The figure shows three views and two pictorial views of one solid part (mm, origin at its lowest corner). Answer the questions. A direction names the side the tool comes from. Give positions to 0.01 mm unless a question says otherwise; leave off trailing zeros. Order: outer loops, then holes, each group sorted by start corner. A loop starts at its lowest first (then second) coordinate and runs counter-clockwise, first axis right, second up. Notation, with made-up numbers: (82.5, -7.5) -> (124.5, -7.5) arc R17 cw to (124.5, 4.5) -> close; hole circle Ø4 at (23, 25.25). An arc over 180 degrees is marked (long way). Use one line per item in the form item = value.
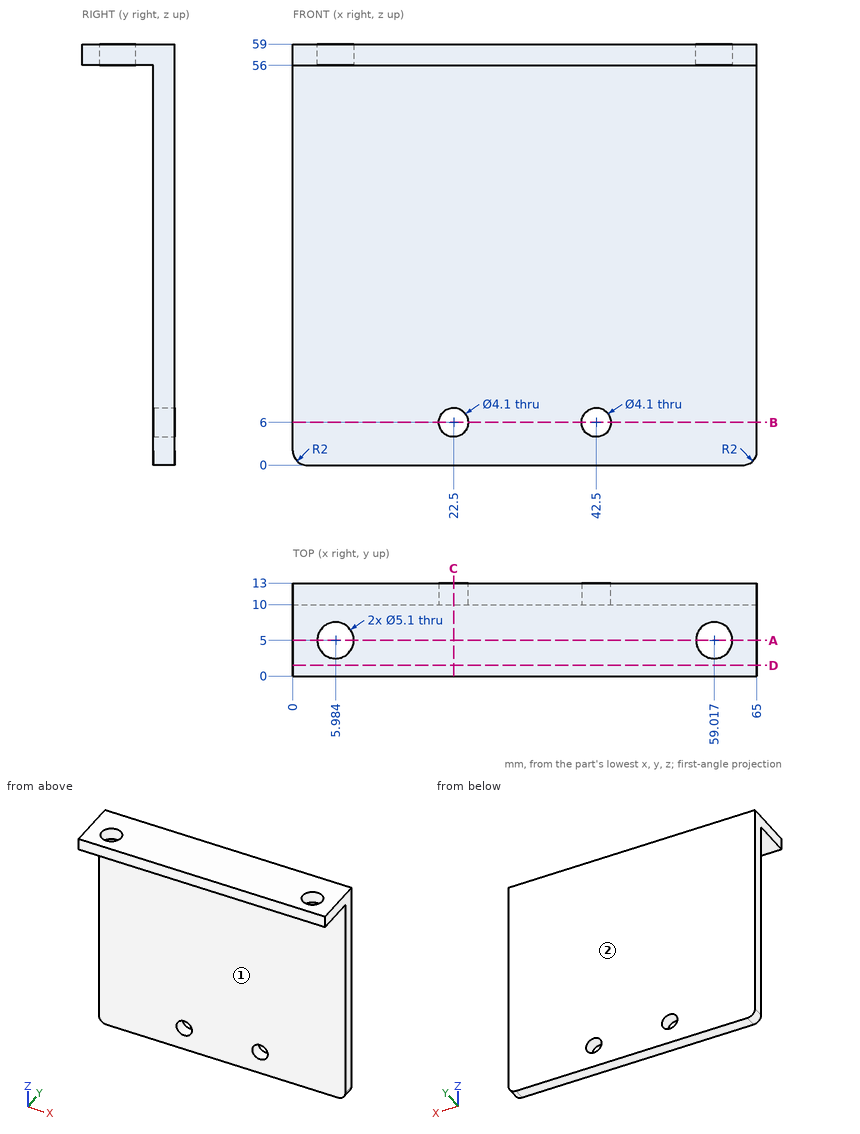
Item 1: The part is cut by section B-B on z = 6. Give the vertices of the cut face in (x, y).
Checks:
outline = (0, 10) -> (20.45, 10) -> (20.45, 13) -> (0, 13) -> close; (24.55, 10) -> (40.45, 10) -> (40.45, 13) -> (24.55, 13) -> close; (44.55, 10) -> (65, 10) -> (65, 13) -> (44.55, 13) -> close
Item 2: Given pin 1 Ø6 at (x, z) = (36.5, 50.5) entering from -Y; pin 2 Ø2 at (x, y) = (26.5, 2) entering from -Z, each flat-ended and moving along its own axis, determine where each tip first touches the part or whether it passes through.
Checks:
pin_1 = 10
pin_2 = 56
Item 3: The part is cut by section D-D on y = 1.5. Give the vertices of the cut face in (x, z).
Checks:
outline = (0, 56) -> (65, 56) -> (65, 59) -> (0, 59) -> close
Item 4: The part is cut by section C-C on x = 22.5. Give the vertices of the cut face in (y, z).
Checks:
outline = (0, 56) -> (10, 56) -> (10, 8.05) -> (13, 8.05) -> (13, 59) -> (0, 59) -> close; (10, 0) -> (13, 0) -> (13, 3.95) -> (10, 3.95) -> close
Item 5: Straight lines are drawn through the part: L1, parallel to Z at x = 22.5, y = 11.5; L2, parallel to Z at x = 40.5, y = 5; L3, parallel to Y at x = 26.5, z = 36.5. For each, find the intervals that lie inside material, in ascending order. Write a range as from..to.
Checks:
L1 = 0..3.95, 8.05..59
L2 = 56..59
L3 = 10..13
Item 6: The part is cut by section A-A on y = 5. Give the vertices of the cut face in (x, z).
Checks:
outline = (0, 56) -> (3.43, 56) -> (3.43, 59) -> (0, 59) -> close; (8.53, 56) -> (56.47, 56) -> (56.47, 59) -> (8.53, 59) -> close; (61.57, 56) -> (65, 56) -> (65, 59) -> (61.57, 59) -> close
Item 7: Which of the six approach directions +Z, -Z, +X, -X, +Y, -Y give full straight-line access (tool end or side, diameter ignored) to the marked faces 1 and 2?
Checks:
face_1 = -Z, +X, -X, -Y
face_2 = +Z, -Z, +X, -X, +Y
